```python
from build123d import *

# Parameters (mm, degrees)
SKETCH_1_W          = 150
SKETCH_1_H          = 100
EXTRUDE_2_DEPTH     = 3
SKETCH_2_R          = 1.5
CUT_EXTRUDE_1_DEPTH = 181.302523554
SKETCH_3_W          = 30
SKETCH_3_H          = 3
CUT_EXTRUDE_2_DEPTH = 181.302523554


with BuildPart() as part:
    # 草图1 → 凸台-拉伸2 (new body)
    with BuildSketch(Plane.XY):
        with Locations((-75, 50)):
            Rectangle(SKETCH_1_W, SKETCH_1_H)
    extrude(amount=EXTRUDE_2_DEPTH)

    # 草图2 → 切除-拉伸1 (cut, through all)
    with BuildSketch(Plane.XY.offset(3)):
        with Locations((-30, 30)):
            Circle(SKETCH_2_R)
        with Locations((-40, 80)):
            Circle(SKETCH_2_R)
    extrude(amount=-CUT_EXTRUDE_1_DEPTH, mode=Mode.SUBTRACT)

    # 草图3 → 切除-拉伸2 (cut, through all)
    with BuildSketch(Plane.XY.offset(3)):
        with Locations((-110, 60)):
            Rectangle(SKETCH_3_W, SKETCH_3_H)
    extrude(amount=-CUT_EXTRUDE_2_DEPTH, mode=Mode.SUBTRACT)


solid = part.part
```
Could you check a few things on this model? Use its own coordinates, in mm. A direction names the side the tool comes from. Give positions to 0.01 mm unless a question says otherwise; leave off trailing zeros. Order: outer loops, then holes, each group sorted by start corner. A loop starts at its lowest first (then second) coordinate and runs counter-clockwise, first axis right, second up.
Q1. I'm going to push a flat-ended pin straight in: P1, Ø2.5, axis at x = -30, y = 30, coming from the +Z side. Where does the tip first touch, or does it pass through?
Q2. For faces 5 (the flat face through (-76, 0, 1)), 6 (the flat face through (-110, 58.5, 2)), which set-ups out of +Z, -Z, +X, -X, +Y, -Y let a thin tool reach every point of the face, with its end or its side?
Q3. We'd pull the mould along X, two halves only. Please class faces 1 (the flat face through (-76, 51, 3)), 2 (the cylindrical face through (-31.5, 30.07, 1.52)), 3 (the cylindrical face through (-41.11, 81.01, 1.52)), 4 (the flat face through (-150, 49, 1)): +X half, -X half, draft (parallel to the pull), parting line (faces both ways), or undercut.
Q4. If I drill on line 1 along X through (y, z) = (80, 1.45); line 2 along Y through (x, z) = (-40, 2.3); line 3 along Y through (x, z) = (-30, 1.15), over which ranges is the centre line in solid material (lowest first)?
Q5. Suppose I cut it at B-B, the plane x = -99. Write out the boundary of the cut face in (y, z).
Q6. Suppose I cut it at A-A, the plane y = 80. Write out the boundary of the cut face in (x, z).
Solution:
1. P1: passes through
2. face 5: +Z, -Z, +X, -X, -Y
2. face 6: +Z, -Z
3. face 1: draft
3. face 2: undercut
3. face 3: undercut
3. face 4: -X half
4. line 1: x = -150 to -41.5, -38.5 to 0
4. line 2: y = 0 to 78.5, 81.5 to 100
4. line 3: y = 0 to 28.5, 31.5 to 100
5. outline: (0, 0) - (58.5, 0) - (58.5, 3) - (0, 3) - close; (61.5, 0) - (100, 0) - (100, 3) - (61.5, 3) - close
6. outline: (-150, 0) - (-41.5, 0) - (-41.5, 3) - (-150, 3) - close; (-38.5, 0) - (0, 0) - (0, 3) - (-38.5, 3) - close
